```python
from build123d import *

# Parameters (mm, degrees)
SKETCH2_R           = 7.9375
SKETCH2_R_2         = 3.175
BOSS_EXTRUDE1_DEPTH = 139.7
SKETCH3_OUTSIDE_W   = 46.174
SKETCH3_OUTSIDE_H   = 46.174
SKETCH3_OUTSIDE_R   = 5.5245
CUT_EXTRUDE1_DEPTH  = 19.05
SKETCH4_OUTSIDE_W   = 46.174
SKETCH4_OUTSIDE_H   = 46.174
SKETCH4_OUTSIDE_R   = 6.35
CUT_EXTRUDE2_DEPTH  = 114.3


with BuildPart() as part:
    # Sketch2 → Boss-Extrude1 (new body)
    with BuildSketch(Plane.XY):
        Circle(SKETCH2_R)
        Circle(SKETCH2_R_2, mode=Mode.SUBTRACT)
    extrude(amount=BOSS_EXTRUDE1_DEPTH)

    # Sketch3 outside → Cut-Extrude1 (cut)
    with BuildSketch(Plane(origin=(0, 0, 0), x_dir=(-1, 0, 0), z_dir=(0, 0, -1))):
        Rectangle(SKETCH3_OUTSIDE_W, SKETCH3_OUTSIDE_H)
        Circle(SKETCH3_OUTSIDE_R, mode=Mode.SUBTRACT)
    extrude(amount=-CUT_EXTRUDE1_DEPTH, mode=Mode.SUBTRACT)

    # Sketch4 outside → Cut-Extrude2 (cut)
    with BuildSketch(Plane.XY.offset(139.7)):
        Rectangle(SKETCH4_OUTSIDE_W, SKETCH4_OUTSIDE_H)
        Circle(SKETCH4_OUTSIDE_R, mode=Mode.SUBTRACT)
    extrude(amount=-CUT_EXTRUDE2_DEPTH, mode=Mode.SUBTRACT)

    # Sketch9 → Cut-Revolve1 (revolve, cut)
    with BuildSketch(Plane(origin=(0, 0, 0), x_dir=(0, 0, -1), z_dir=(1, 0, 0)), mode=Mode.PRIVATE) as cut_revolve1_sk:
        Polygon((-133.985, 4.7244), (-139.7, 4.224402288), (-139.7, 6.35), (-128.27, 6.35), (-128.27, 4.572), (-130.048, 4.572), (-130.048, 5.3975), (-133.3119, 5.3975), align=None)
    revolve(cut_revolve1_sk.sketch.rotate(Axis((0, 0, 139.7), (0, 0, -1)), 90), axis=Axis((0, 0, 139.7), (0, 0, -1)), mode=Mode.SUBTRACT)


solid = part.part
```
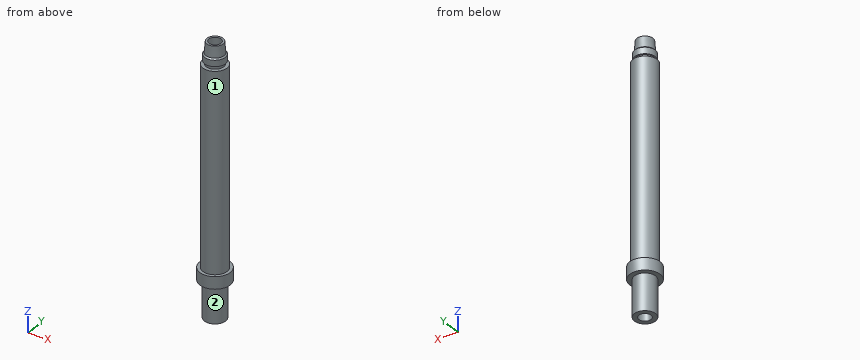
CAD build for the part. Positions are in the model's coordinates, mm. Face numbers are marked on the shaded views. A direction names the side the tool comes from. Round coordinates to 2 decimals unless told otherwise and drop trailing zeros. Order: outer loops, then holes, each group sorted by start corner. A loop starts at its lowest first (then second) coordinate and runs counter-clockwise, first axis right, second up.
Item 1: Pin check, flat tips, straight feed: pin 1 (5 mm diameter, centred on x = -3, z = 53, fed in from +Y); pin 2 (3 mm diameter, centred on x = -5.5, z = 60, fed in from -Y); pin 3 (1 mm diameter, centred on x = -4, y = 1.5, fed in from +Z); pin 4 (5 mm diameter, centred on y = 3.5, z = 59, fed in from +X). Stop position of each tip, or through.
Item 2: Saw through at D-D on z = 113. Write the cut outline in (x, y) (3 decimals).
Item 3: Probe line 1 along Y through (x, z) = (0, 79.5) (3 decimals); line 2 along Z through (x, y) = (4, -5.25); line 3 along X through (y, z) = (0.25, 100.5). List the from-to ranges inside material, lowest first.
Item 4: Tool access for the marked faces 1 and 2: list every direction of +Z, -Z, +X, -X, +Y, -Y with a clear straight run to the whole face (end or side of a thin tool).
Reported:
1. pin 1: stops at y = 6.33
1. pin 2: stops at y = -4.93
1. pin 3: stops at z = 139.7
1. pin 4: stops at x = 6.27
2. outline: circle Ø12.7 at (0, 0); hole circle Ø6.35 at (0, 0)
3. line 1: y = -6.35 to -3.175, 3.175 to 6.35
3. line 2: z = 19.05 to 25.4
3. line 3: x = -6.35 to -3.17, 3.17 to 6.35
4. face 1: +Z
4. face 2: -Z
